from build123d import *

# Parameters (mm, degrees)
SKETCH_1_R          = 5
EXTRUDE_1_DEPTH     = 10
SKETCH_2_R          = 10
SKETCH_2_R_2        = 5
EXTRUDE_2_DEPTH     = 16
SKETCH_3_R          = 7.5
CUT_EXTRUDE_1_DEPTH = 10
SKETCH_4_R          = 18.5
CUT_EXTRUDE_2_DEPTH = 10
SKETCH_5_R          = 18.5
SKETCH_5_R_2        = 10.1
EXTRUDE_3_DEPTH     = 2


with BuildPart() as part:
    # 草图1 → 凸台-拉伸1 (new body)
    with BuildSketch(Plane.XY):
        with BuildLine():
            ThreePointArc((-128.022678922, -73.913928138), (-90.421378279, 38.440519474), (0, 115))
            ThreePointArc((0, 115), (90.421378279, 38.440519474), (128.022678922, -73.913928138))
            ThreePointArc((128.022678922, -73.913928138), (0, -115), (-128.022678922, -73.913928138))
        make_face()
        with Locations((0, 103)):
            Circle(SKETCH_1_R, mode=Mode.SUBTRACT)
        with Locations((-117.630374076, -67.913928138)):
            Circle(SKETCH_1_R, mode=Mode.SUBTRACT)
        with Locations((117.630374076, -67.913928138)):
            Circle(SKETCH_1_R, mode=Mode.SUBTRACT)
    extrude(amount=EXTRUDE_1_DEPTH)

    # 草图2 → 凸台-拉伸2 (add)
    # profile 1 of 3: a face of its own
    with BuildSketch(Plane.XY.offset(10)):
        with Locations((0, 103)):
            Circle(SKETCH_2_R)
        with Locations((0, 103)):
            Circle(SKETCH_2_R_2, mode=Mode.SUBTRACT)
    # profile 2 of 3: a face of its own
    with BuildSketch(Plane.XY.offset(10)):
        with Locations(Location((-117.630374076, -67.913928138, 0), (0, 0, 179.375778052))):
            Circle(SKETCH_2_R)
        with Locations((-117.630374076, -67.913928138)):
            Circle(SKETCH_2_R_2, mode=Mode.SUBTRACT)
    # profile 3 of 3: a face of its own
    with BuildSketch(Plane.XY.offset(10)):
        with Locations(Location((117.630374076, -67.913928138, 0), (0, 0, 8.696571879))):
            Circle(SKETCH_2_R)
        with Locations((117.630374076, -67.913928138)):
            Circle(SKETCH_2_R_2, mode=Mode.SUBTRACT)
    extrude(amount=EXTRUDE_2_DEPTH)

    # 草图3 → 切除-拉伸1 (cut)
    with BuildSketch(Plane(origin=(0, 0, 0), x_dir=(-1, 0, 0), z_dir=(0, 0, -1))):
        with Locations((12.650995066, 69.515536741)):
            Circle(SKETCH_3_R)
        with Locations((82.334125615, -39.530718783)):
            Circle(SKETCH_3_R)
    extrude(amount=-CUT_EXTRUDE_1_DEPTH, mode=Mode.SUBTRACT)

    # 草图4 → 切除-拉伸2 (cut)
    with BuildSketch(Plane.XY.offset(10)):
        with Locations((12.425309319, -23.296523673)):
            Circle(SKETCH_4_R)
    extrude(amount=-CUT_EXTRUDE_2_DEPTH, mode=Mode.SUBTRACT)

    # 草图5 → 凸台-拉伸3 (add)
    with BuildSketch(Plane.XY.offset(10)):
        with Locations((12.425309319, -23.296523673)):
            Circle(SKETCH_5_R)
        with Locations((12.425309319, -23.296523673)):
            Circle(SKETCH_5_R_2, mode=Mode.SUBTRACT)
    extrude(amount=-EXTRUDE_3_DEPTH)


solid = part.part
Verification items for the finished model (mm, model axes). A direction names the side the tool comes from. Coordinates: 2 decimals unless noted, no trailing zeros. Order: outer loops, then holes, each group sorted by start corner. A loop starts at its lowest first (then second) coordinate and runs counter-clockwise, first axis right, second up. Notation, with made-up numbers: (44, 83) -> (67, 83) arc R25 cw to (67, 95) -> close; hole circle Ø6 at (-2.75, 71.25). An arc over 180 degrees is marked (long way). Put each result on its own line as item: value. Start each with the question number.
1. Material ranges on L1, parallel to Y at x = 0, z = 17.75; L2, parallel to Z at x = 78, y = 27; L3, parallel to Y at x = 0, z = 5.5, recorded low to high. Write a range as [from, to].
2. Cross-section at D-D, the plane y = 33. Record the boundary of the cut face in (x, z).
3. Cross-section at A-A, the plane z = 4.5. Record the boundary of the cut face in (x, y).
4. Cross-section at C-C, the plane x = 79. Record the boundary of the cut face in (y, z), then the cut area to 3 significant figures.
5. Go/stop test with flat-tipped pins: pin 1 Ø6 at (x, z) = (-32.5, 5) entering from -Y; pin 2 Ø6 at (x, y) = (15, 51.5) entering from +Z; pin 3 Ø2 at (y, z) = (90, 5) entering from +X; pin 4 Ø12 at (x, y) = (31.5, -62.5) entering from -Z. Record where each tip stops, or that it passes through.
6. Cross-section at B-B, the plane y = 103. Record the boundary of the cut face in (x, z), then the cut area to 3 significant figures.
7. Mould release check, pull along Y, two halves, no side actions. Record for faces 4 (the cylindrical face through (-19.58, 66.64, 4.93)), 5 (the flat face through (-2, -24, 10)), 6 (the cylindrical face through (-91.358, 37.047, 4.93)): released by +Y, released by -Y, zero draft, split by the parting line, or undercut.
8. Access from +Z, -Z, +X, -X, +Y, -Y to the whole of each face (thin tool, end or side, straight path). Record for faces 1 (the cylindrical face through (22.371, -7.697, 4.056)), 2 (the cylindrical face through (-110.33, -74.75, 17.89)), 3 (the cylindrical face through (-1.08, 98.12, 12.82)).
Computed:
1. L1: [93, 98], [108, 113]
1. L2: [0, 10]
1. L3: [-115, -37], [-9.59, 98], [108, 115]
2. outline: (-93.99, 0) -> (93.99, 0) -> (93.99, 10) -> (-93.99, 10) -> close
3. outline: (-128.02, -73.91) arc R220 ccw to (128.02, -73.91) arc R220 ccw to (0, 115) arc R220 ccw to start; hole circle Ø10 at (-117.63, -67.91); hole circle Ø15 at (-82.33, -39.53); hole circle Ø15 at (-12.65, 69.52); hole circle Ø37 at (12.43, -23.3); hole circle Ø10 at (0, 103); hole circle Ø10 at (117.63, -67.91)
4. outline: (-100.33, 0) -> (53.81, 0) -> (53.81, 10) -> (-100.33, 10) -> close
4. area: 1,540 mm2
5. pin 1: y = -113.01
5. pin 2: z = 10
5. pin 3: x = 42.95
5. pin 4: z = 0
6. outline: (-22.6, 0) -> (-5, 0) -> (-5, 26) -> (-10, 26) -> (-10, 10) -> (-22.6, 10) -> close; (5, 0) -> (22.6, 0) -> (22.6, 10) -> (10, 10) -> (10, 26) -> (5, 26) -> close
6. area: 512 mm2
7. face 4: undercut
7. face 5: zero draft
7. face 6: released by +Y
8. face 1: -Z
8. face 2: +Z
8. face 3: +Z, -Z
